Design review of the part shown in the three views and the two pictorial views. Dimensions are in mm from the part's minimum x, y and z. A direction names the side the tool comes from. Round coordinates to 2 decimals unless told otherwise and drop trailing zeros. Order: outer loops, then holes, each group sorted by start corner. A loop starts at its lowest first (then second) coordinate and runs counter-clockwise, first axis right, second up.
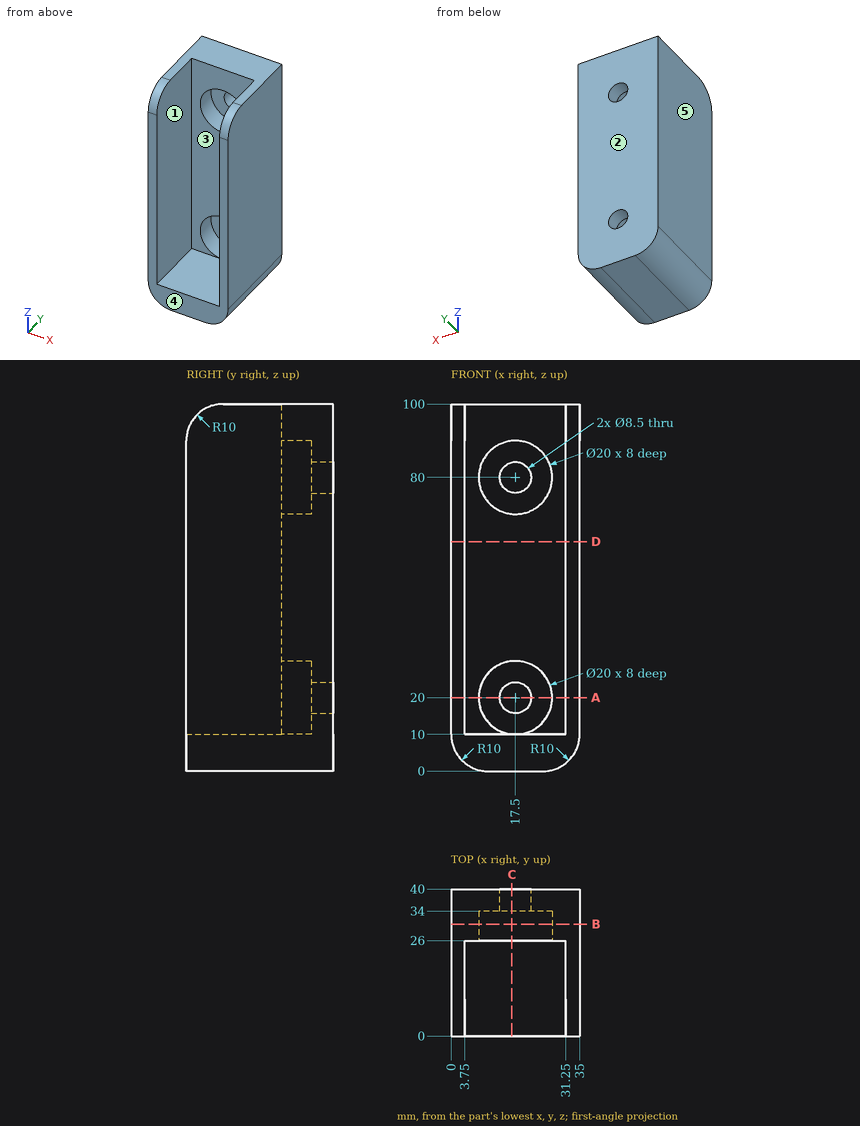
(1) For the marked faces 1 and 2, list the 3-axis set-ups (+Z, -Z, +X, -X, +Y, -Y) from which the entire face can be reached by the end or side of a thin tool; tool diameter is ignored.
Data:
face 1: +Z, -Y
face 2: +Z, -Z, +X, -X, +Y
(2) Consider section A-A (z = 20). Write out the cut boundary in (x, y), and give its area (3 significant figures).
Data:
outline: (0, 0) - (3.75, 0) - (3.75, 26) - (7.5, 26) - (7.5, 34) - (13.25, 34) - (13.25, 40) - (0, 40) - close; (21.75, 34) - (27.5, 34) - (27.5, 26) - (31.25, 26) - (31.25, 0) - (35, 0) - (35, 40) - (21.75, 40) - close
area: 474 mm2
(3) Insertion check: pin 1 (7 mm diameter, centred on x = 17.5, z = 20, fed in from -Y); pin 2 (4 mm diameter, centred on x = 6.5, y = 5, fed in from -Z); pin 3 (6 mm diameter, centred on x = 14, z = 19, fed in from -Y); pin 4 (2 mm diameter, centred on x = 21, y = 10.5, fed in from +Z). Each pin has a flat end and moves straight along its axis. Give the tip position at first contact, or say it passes through.
Data:
pin 1: passes through
pin 2: stops at z = 0.11
pin 3: stops at y = 34
pin 4: stops at z = 10
(4) Consider section D-D (z = 62.5). Write out the cut boundary in (x, y).
Data:
outline: (0, 0) - (3.75, 0) - (3.75, 26) - (31.25, 26) - (31.25, 0) - (35, 0) - (35, 40) - (0, 40) - close
(5) Consider section B-B (y = 30.5). Write out the cut boundary in (x, z).
Data:
outline: (0, 10) arc R10 ccw to (10, 0) - (25, 0) arc R10 ccw to (35, 10) - (35, 100) - (0, 100) - close; hole circle Ø20 at (17.5, 20); hole circle Ø20 at (17.5, 80)
(6) To check wall thickness, follow probe 1 along Z at (x, y) = (17.5, 38.3); probe 2 along Z at (x, y) = (17, 29); probe 3 along X at (y, z) = (15.5, 25.5). State the ranges of each line that lie inside material, in increasing order.
Data:
probe 1: z = 0 to 15.75, 24.25 to 75.75, 84.25 to 100
probe 2: z = 0 to 10.01, 29.99 to 70.01, 89.99 to 100
probe 3: x = 0 to 3.75, 31.25 to 35
(7) Consider section C-C (x = 16.5). Write out the cut boundary in (y, z), and give its area (3 significant figures).
Data:
outline: (0, 0) - (40, 0) - (40, 15.87) - (34, 15.87) - (34, 10.05) - (26, 10.05) - (26, 10) - (0, 10) - close; (26, 29.95) - (34, 29.95) - (34, 24.13) - (40, 24.13) - (40, 75.87) - (34, 75.87) - (34, 70.05) - (26, 70.05) - close; (26, 89.95) - (34, 89.95) - (34, 84.13) - (40, 84.13) - (40, 100) - (26, 100) - close
area: 1,240 mm2
(8) Draft analysis for pull direction X (two halves, no side actions). For the marked faces 3, 4 and 5, state which applies: pulls with the +X half, pulls with the -X half, needs draft (parallel to the pull), parting line crosses it, or undercut.
Data:
face 3: undercut
face 4: needs draft
face 5: pulls with the -X half
